The listing builds one solid part. Answer for the finished solid, in the listing's coordinates (mm). A direction names the side the tool comes from. Coordinates: 2 decimals unless noted, no trailing zeros. Order: outer loops, then holes, each group sorted by start corner. A loop starts at its lowest first (then second) coordinate and runs counter-clockwise, first axis right, second up. Notation, with made-up numbers: (54, 39) -> (90, 39) arc R19 cw to (90, 70) -> close; hole circle Ø5 at (7, 61.25). An arc over 180 degrees is marked (long way). Return JSON: item names as keys, results as strings.
```python
from build123d import *

# Parameters (mm, degrees)
ESQUISSE1_W             = 160
ESQUISSE1_H             = 90
EXTRUSION1_DEPTH        = 50
CONG_1_R                = 25
CONG_2_R                = 15
COQUE1_T                = -4
ESQUISSE2_W             = 50
ESQUISSE2_H             = 15
ENL_V_MAT_EXTRU_1_DEPTH = 3
CONG_4_R                = 3
CONG_5_R                = 3
CONG_6_R                = 3
CONG_7_R                = 3
CONG_4_OF_SYM_TRIE1_R   = 3
CONG_5_OF_SYM_TRIE1_R   = 3
CONG_6_OF_SYM_TRIE1_R   = 3
CONG_7_OF_SYM_TRIE1_R   = 3


with BuildPart() as part:
    # Esquisse1 → Extrusion1 (new body)
    with BuildSketch(Plane(origin=(0, 0, 0), x_dir=(1, 0, 0), z_dir=(0, 1, 0))):
        with Locations((35.341232877, 23.705753425)):
            Rectangle(ESQUISSE1_W, ESQUISSE1_H)
    extrude(amount=EXTRUSION1_DEPTH)

    # Congé1
    cong_1_edges = [part.edges().sort_by_distance(p)[0] for p in [
        (115.341232877, 50, -23.705753425),
        (-44.658767123, 50, -23.705753425),
    ]]
    fillet(cong_1_edges, radius=CONG_1_R)

    # Congé2
    cong_2_edges = [part.edges().sort_by_distance(p)[0] for p in [
        (35.341232877, 50, 21.294246575),
        (35.341232877, 50, -68.705753425),
        (115.341232877, 12.5, 21.294246575),
        (-44.658767123, 12.5, 21.294246575),
        (108.018902406, 42.67766953, 21.294246575),
        (-37.336436653, 42.67766953, 21.294246575),
        (-44.658767123, 12.5, -68.705753425),
        (115.341232877, 12.5, -68.705753425),
        (108.018902406, 42.67766953, -68.705753425),
        (-37.336436653, 42.67766953, -68.705753425),
    ]]
    fillet(cong_2_edges, radius=CONG_2_R)

    # Coque1
    coque1_openings = [part.faces().sort_by_distance(p)[0] for p in [
        (35.341232877, 0, -23.705753425),
    ]]
    offset(amount=COQUE1_T, openings=coque1_openings, kind=Kind.INTERSECTION)

    # Esquisse2 → Enlèv. mat.-Extru.1 (cut)
    with BuildSketch(Plane.XY.offset(21.294246575)):
        with Locations((35.341232877, 22.5)):
            Rectangle(ESQUISSE2_W, ESQUISSE2_H)
    enl_v_mat_extru_1 = extrude(amount=-ENL_V_MAT_EXTRU_1_DEPTH, mode=Mode.SUBTRACT)

    # Congé4
    cong_4_edges = [part.edges().sort_by_distance(p)[0] for p in [
        (35.341232877, 15, 18.294246575),
    ]]
    fillet(cong_4_edges, radius=CONG_4_R - 0.0001)  # a hair under: the kernel refuses the full size

    # Congé5
    cong_5_edges = [part.edges().sort_by_distance(p)[0] for p in [
        (35.341232877, 30, 18.294246575),
    ]]
    fillet(cong_5_edges, radius=CONG_5_R - 0.0001)  # a hair under: the kernel refuses the full size

    # Congé6
    cong_6_edges = [part.edges().sort_by_distance(p)[0] for p in [
        (10.341232877, 15.878650367, 19.172896942),
        (10.341232877, 22.5, 18.294246575),
        (10.341232877, 29.121349633, 19.172896942),
    ]]
    fillet(cong_6_edges, radius=CONG_6_R - 0.0001)  # a hair under: the kernel refuses the full size

    # Congé7
    cong_7_edges = [part.edges().sort_by_distance(p)[0] for p in [
        (60.341232877, 22.5, 18.294246575),
        (60.341232877, 15.878650367, 19.172896942),
        (60.341232877, 29.121349633, 19.172896942),
    ]]
    fillet(cong_7_edges, radius=CONG_7_R - 0.0001)  # a hair under: the kernel refuses the full size

    # Symétrie1: Enlèv. mat.-Extru.1 across plane
    add(enl_v_mat_extru_1.mirror(Plane.XY.offset(-23.705753425)), mode=Mode.SUBTRACT)

    # Congé4 of Symétrie1
    cong_4_of_sym_trie1_edges = [part.edges().sort_by_distance(p)[0] for p in [
        (35.341232877, 15, -65.705753425),
    ]]
    fillet(cong_4_of_sym_trie1_edges, radius=CONG_4_OF_SYM_TRIE1_R - 0.0001)  # a hair under: the kernel refuses the full size

    # Congé5 of Symétrie1
    cong_5_of_sym_trie1_edges = [part.edges().sort_by_distance(p)[0] for p in [
        (35.341232877, 30, -65.705753425),
    ]]
    fillet(cong_5_of_sym_trie1_edges, radius=CONG_5_OF_SYM_TRIE1_R - 0.0001)  # a hair under: the kernel refuses the full size

    # Congé6 of Symétrie1
    cong_6_of_sym_trie1_edges = [part.edges().sort_by_distance(p)[0] for p in [
        (10.341232877, 15.878650367, -66.584403792),
        (10.341232877, 22.5, -65.705753425),
        (10.341232877, 29.121349633, -66.584403792),
    ]]
    fillet(cong_6_of_sym_trie1_edges, radius=CONG_6_OF_SYM_TRIE1_R - 0.0001)  # a hair under: the kernel refuses the full size

    # Congé7 of Symétrie1
    cong_7_of_sym_trie1_edges = [part.edges().sort_by_distance(p)[0] for p in [
        (60.341232877, 22.5, -65.705753425),
        (60.341232877, 15.878650367, -66.584403792),
        (60.341232877, 29.121349633, -66.584403792),
    ]]
    fillet(cong_7_of_sym_trie1_edges, radius=CONG_7_OF_SYM_TRIE1_R - 0.0001)  # a hair under: the kernel refuses the full size


solid = part.part
```
Item 1: Find the intervals of material crossed by probe 1 along Z at (x, y) = (18.5, 13); probe 2 along X at (y, z) = (12, -45.5); probe 3 along Y at (x, z) = (23, 2), in increasing order.
Answer list:
{"probe 1": "-68.71 to -64.71, 17.29 to 21.29", "probe 2": "-44.66 to -40.66, 111.34 to 115.34", "probe 3": "46 to 50"}
Item 2: The part is cut by section C-C on z = -31. Determine the outline of the cut face in (x, y), plus the area to 3 significant figures.
Answer list:
{"outline": "(-44.66, 0) -> (-40.66, 0) -> (-40.66, 25) arc R21 cw to (-19.66, 46) -> (90.34, 46) arc R21 cw to (111.34, 25) -> (111.34, 0) -> (115.34, 0) -> (115.34, 25) arc R25 ccw to (90.34, 50) -> (-19.66, 50) arc R25 ccw to (-44.66, 25) -> close", "area": "929 mm2"}
Item 3: The part is cut by section D-D on x = 3. Determine the outline of the cut face in (y, z).
Answer list:
{"outline": "(0, -68.71) -> (35, -68.71) arc R15 ccw to (50, -53.71) -> (50, 6.29) arc R15 ccw to (35, 21.29) -> (0, 21.29) -> (0, 17.29) -> (35, 17.29) arc R11 cw to (46, 6.29) -> (46, -53.71) arc R11 cw to (35, -64.71) -> (0, -64.71) -> close"}
Item 4: Flat-ended cylindrical pins translate along their axes: pin 1 (2.5 mm diameter, centred on x = 25, y = 24.5, fed in from +Z); pin 2 (3 mm diameter, centred on x = -23, z = -1.5, fed in from +Y); pin 3 (1 mm diameter, centred on x = 43.5, z = -15, fed in from -Y). Find the tip coordinate at first contact, or state that the pin passes through.
Answer list:
{"pin 1": "z = 18.29", "pin 2": "y = 49.93", "pin 3": "y = 46"}
Item 5: Determine the mould class of faces 1 (the cylindrical face through (36.11, 42.69, -61.57)), 2 (the cylindrical face through (-40.148, 12.675, -64.428)), 3 (the flat face through (35, 0, 19)) for opening direction Z: pulls with the +Z half, pulls with the -Z half, needs draft (parallel to the pull), parting line crosses it, or undercut.
Answer list:
{"face 1": "undercut", "face 2": "pulls with the -Z half", "face 3": "needs draft"}
Item 6: Which of the six approach directions +Z, -Z, +X, -X, +Y, -Y give full straight-line access (tool end or side, diameter ignored) to faces 4 (the flat face through (35, 50, -24)), 5 (the cylindrical face through (36.11, 42.69, 14.16)), 6 (the cylindrical face through (59.49, 22.56, -66.61)), 7 (the cylindrical face through (36.11, 45.49, -64.43)), 8 (the flat face through (35, 23, 18.294))?
Answer list:
{"face 4": "+Z, -Z, +X, -X, +Y", "face 5": "-Y", "face 6": "-Z", "face 7": "-Z, +X, -X, +Y", "face 8": "+Z"}
